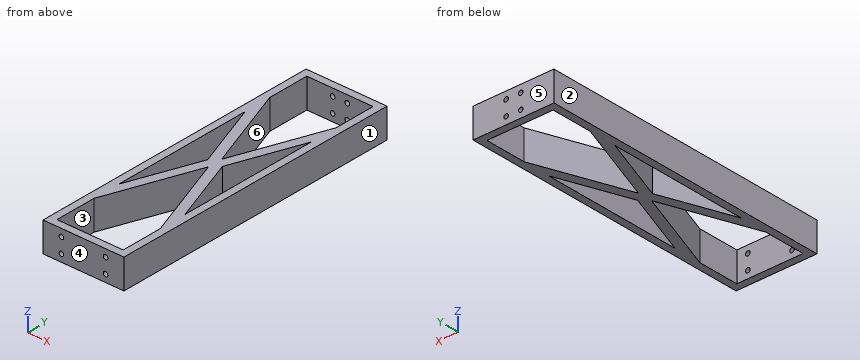
from build123d import *

# Parameters (mm, degrees)
SKETCH_W        = 55
SKETCH_H        = 200
PAD_DEPTH       = 20
POCKET_DEPTH    = 20
SKETCH002_R     = 1.55
POCKET001_DEPTH = 5
SKETCH003_R     = 1.55
POCKET002_DEPTH = 5


with BuildPart() as part:
    # Sketch → Pad (new body)
    with BuildSketch(Plane.XY):
        Rectangle(SKETCH_W, SKETCH_H)
    extrude(amount=PAD_DEPTH)

    # Sketch001 (on Face6 of Pad) → Pocket (cut)
    with BuildSketch(Plane.XY.offset(20)):
        Polygon((-22.5, -95), (22.5, -95), (22.5, -66.818242), (0, -5), (-22.5, -66.818242), align=None)
        Polygon((-22.5, 95), (22.5, 95), (22.5, 66.818242), (0, 5), (-22.5, 66.818242), align=None)
        Polygon((-5, 0), (-22.5, -48.080855), (-22.5, 48.080855), align=None)
        Polygon((5, 0), (22.5, 48.080855), (22.5, -48.080855), align=None)
    extrude(amount=-POCKET_DEPTH, mode=Mode.SUBTRACT)

    # Sketch002 (on Face3 of Pocket) → Pocket001 (cut)
    with BuildSketch(Plane(origin=(0, 100, 0), x_dir=(-1, 0, 0), z_dir=(0, 1, 0))):
        with Locations((-5, 15)):
            Circle(SKETCH002_R)
        with Locations((5, 15)):
            Circle(SKETCH002_R)
        with Locations((5, 5)):
            Circle(SKETCH002_R)
        with Locations((-5, 5)):
            Circle(SKETCH002_R)
    extrude(amount=-POCKET001_DEPTH, mode=Mode.SUBTRACT)

    # Sketch003 (on Face2 of Pocket001) → Pocket002 (cut)
    with BuildSketch(Plane.XZ.offset(100)):
        with Locations((-15, 15)):
            Circle(SKETCH003_R)
        with Locations((15, 15)):
            Circle(SKETCH003_R)
        with Locations((15, 5)):
            Circle(SKETCH003_R)
        with Locations((-15, 5)):
            Circle(SKETCH003_R)
    extrude(amount=-POCKET002_DEPTH, mode=Mode.SUBTRACT)


solid = part.part
The model under review builds one solid part; all positions refer to its coordinate system, in mm. Face numbers are marked on the shaded views. A direction names the side the tool comes from. Give positions to 0.01 mm unless a question says otherwise; leave off trailing zeros. Order: outer loops, then holes, each group sorted by start corner. A loop starts at its lowest first (then second) coordinate and runs counter-clockwise, first axis right, second up. Notation, with made-up numbers: (-13.5, 22.25) -> (10.5, 22.25) arc R6 ccw to (10.5, 30.25) -> close; hole circle Ø5 at (-39.75, 14.25). An arc over 180 degrees is marked (long way). Write item = value, one per line. Start each with the question number.
(1) Take a section at A-A (x = 10.5). Write out the cut boundary in (y, z), plus the area to 3 significant figures.
(2) Tool access review of the marked faces 5 and 6: name each direction out of +Z, -Z, +X, -X, +Y, -Y from which nothing blocks a thin tool from reaching the whole face with its end or side.
(3) For pin 1 Ø6 at (x, y) = (-17.5, 14) entering from +Z, flat-tipped, find the tip position at first contact; note if it passes through.
(4) For L1, parallel to Z at x = 15, y = -97; L2, parallel to X at y = -70.5, z = 15.5; L3, parallel to X at y = 46.5, z = 6, list the stretches that pass through material, from the lowest coordinate up. Write a range as from..to.
(5) Take a section at B-B (y = -61). Write out the cut boundary in (x, z).
(6) Draft analysis for pull direction X (two halves, no side actions). For the marked faces 1, 2, 3 and 4, state which applies: +X half, -X half, draft (parallel to the pull), parting line (faces both ways), or undercut.
(7) Take a section at C-C (y = 38.5). Write out the cut boundary in (x, z), plus the area to 3 significant figures.
Returned:
q1.outline = (-100, 0) -> (-95, 0) -> (-95, 20) -> (-100, 20) -> close; (-33.85, 0) -> (-15.11, 0) -> (-15.11, 20) -> (-33.85, 20) -> close; (15.11, 0) -> (33.85, 0) -> (33.85, 20) -> (15.11, 20) -> close; (95, 0) -> (100, 0) -> (100, 20) -> (95, 20) -> close
q1.area = 949 mm²
q2.face_5 = +Z, -Z, +X, -X, +Y
q2.face_6 = +Z, -Z
q3.pin_1 = through
q4.L1 = 0..3.45, 6.55..13.45, 16.55..20
q4.L2 = -27.5..-22.5, 22.5..27.5
q4.L3 = -27.5..-22.5, -21.92..-15.1, 15.1..21.92, 22.5..27.5
q5.outline = (-27.5, 0) -> (-20.38, 0) -> (-20.38, 20) -> (-27.5, 20) -> close; (20.38, 0) -> (27.5, 0) -> (27.5, 20) -> (20.38, 20) -> close
q6.face_1 = +X half
q6.face_2 = -X half
q6.face_3 = undercut
q6.face_4 = draft
q7.outline = (-27.5, 0) -> (-22.5, 0) -> (-22.5, 20) -> (-27.5, 20) -> close; (-19.01, 0) -> (-12.19, 0) -> (-12.19, 20) -> (-19.01, 20) -> close; (12.19, 0) -> (19.01, 0) -> (19.01, 20) -> (12.19, 20) -> close; (22.5, 0) -> (27.5, 0) -> (27.5, 20) -> (22.5, 20) -> close
q7.area = 473 mm²
